from build123d import *

# Parameters (mm, degrees)
EXTRUDE_1_DEPTH     = 10
CUT_EXTRUDE_1_REACH = 177.427
SKETCH_2_R          = 2.15
FILLET_1_R          = 0.6


with BuildPart() as part:
    # 草图1 → 凸台-拉伸1 (new body)
    with BuildSketch(Plane(origin=(0, 0, 0), x_dir=(1, 0, 0), z_dir=(0, 1, 0))):
        with BuildLine():
            Line((-19, 0), (19, 0))
            Line((19, 0), (44.854614973, 30.81233028))
            ThreePointArc((44.854614973, 30.81233028), (46.529317931, 33.929104052), (46.82231051, 37.455159084))
            Line((46.82231051, 37.455159084), (33.389549678, 146.856216784))
            ThreePointArc((33.389549678, 146.856216784), (34.753999407, 148.533855984), (36.376927445, 147.104765038))
            ThreePointArc((36.376927445, 147.104765038), (36.892496808, 144.296291333), (37.320815542, 141.473193853))
            Line((37.320815542, 141.473193853), (37.815132232, 139.258398169))
            ThreePointArc((37.815132232, 139.258398169), (37.817176658, 139.245056143), (37.817405692, 139.231560332))
            Line((37.817405692, 139.231560332), (37.557917484, 134.104765038))
            ThreePointArc((37.557917484, 134.104765038), (40.754926912, 130.959847465), (43.503129215, 134.503681536))
            Line((43.503129215, 134.503681536), (43.077003941, 137.813685213))
            Line((43.077003941, 137.813685213), (42.807637334, 138.925557366))
            ThreePointArc((42.807637334, 138.925557366), (42.806315787, 138.931905108), (42.80540838, 138.938325149))
            Line((42.80540838, 138.938325149), (42.129277547, 145.175318139))
            Line((42.129277547, 145.175318139), (41.965181023, 146.44996701))
            ThreePointArc((41.965181023, 146.44996701), (43.130662006, 148.010841711), (44.727999785, 146.895858405))
            Line((44.727999785, 146.895858405), (66.016482503, 37.376109146))
            ThreePointArc((66.016482503, 37.376109146), (66.063066684, 33.817543133), (64.860464706, 30.468019192))
            Line((64.860464706, 30.468019192), (38.23055697, -15.656334008))
            ThreePointArc((38.23055697, -15.656334008), (35.050772773, -18.836118205), (30.707106781, -20))
            Line((30.707106781, -20), (5.707106781, -20))
            ThreePointArc((5.707106781, -20), (5.515765065, -19.961939766), (5.353553391, -19.853553391))
            Line((5.353553391, -19.853553391), (5, -19.5))
            Line((5, -19.5), (-5, -19.5))
            Line((-5, -19.5), (-5.353553391, -19.853553391))
            ThreePointArc((-5.353553391, -19.853553391), (-5.515765065, -19.961939766), (-5.707106781, -20))
            Line((-5.707106781, -20), (-25.399802658, -20))
            ThreePointArc((-25.399802658, -20), (-30.087775174, -18.833058003), (-33.681629288, -15.604582738))
            Line((-33.681629288, -15.604582738), (-64.860464706, 30.468019192))
            ThreePointArc((-64.860464706, 30.468019192), (-66.063066684, 33.817543133), (-66.016482503, 37.376109146))
            Line((-66.016482503, 37.376109146), (-46.829620455, 141.890886738))
            ThreePointArc((-46.829620455, 141.890886738), (-43.465252598, 152.148967586), (-37.480163066, 161.13372674))
            ThreePointArc((-37.480163066, 161.13372674), (-33.620696298, 161.680216975), (-32.479267504, 157.953116813))
            ThreePointArc((-32.479267504, 157.953116813), (-35.579400499, 146.14570295), (-34.973851142, 133.953116813))
            Line((-34.973851142, 133.953116813), (-47.176674229, 34.569098196))
            ThreePointArc((-47.176674229, 34.569098196), (-47.109221395, 33.75732882), (-46.723670812, 33.03978429))
            Line((-46.723670812, 33.03978429), (-19, 0))
        make_face()
    extrude(amount=EXTRUDE_1_DEPTH)

    # 草图2 → 切除-拉伸1 (cut, up to next)
    with BuildSketch(Plane(origin=(0, 10, 0), x_dir=(1, 0, 0), z_dir=(0, 1, 0)), mode=Mode.PRIVATE) as cut_extrude_1_sk1:
        with Locations(Location((0, -15.5, 0), (0, 0, 270))):
            Circle(SKETCH_2_R)
    cut_extrude_1_tool1 = extrude(cut_extrude_1_sk1.sketch, amount=-CUT_EXTRUDE_1_REACH, mode=Mode.PRIVATE) & part.part
    # 草图2 → 切除-拉伸1 (cut, up to next)
    with BuildSketch(Plane(origin=(0, 10, 0), x_dir=(1, 0, 0), z_dir=(0, 1, 0)), mode=Mode.PRIVATE) as cut_extrude_1_sk2:
        with Locations(Location((0, -7.5, 0), (0, 0, 270))):
            Circle(SKETCH_2_R)
    cut_extrude_1_tool2 = extrude(cut_extrude_1_sk2.sketch, amount=-CUT_EXTRUDE_1_REACH, mode=Mode.PRIVATE) & part.part
    # 草图2 → 切除-拉伸1 (cut, up to next)
    with BuildSketch(Plane(origin=(0, 10, 0), x_dir=(1, 0, 0), z_dir=(0, 1, 0)), mode=Mode.PRIVATE) as cut_extrude_1_sk3:
        with BuildLine():
            Line((-36.549558395, 121.120011078), (-38.607748185, 104.35740041))
            ThreePointArc((-38.607748185, 104.35740041), (-42.47341142, 116.594845153), (-44.332546284, 129.292956179))
            Line((-44.332546284, 129.292956179), (-43.845113062, 129.987442667))
            ThreePointArc((-43.845113062, 129.987442667), (-43.702378092, 130.509625408), (-43.924830211, 131.003146575))
            Line((-43.924830211, 131.003146575), (-44.447419993, 131.543571067))
            ThreePointArc((-44.447419993, 131.543571067), (-44.482588605, 132.737575539), (-44.499925482, 133.931972015))
            ThreePointArc((-44.499925482, 133.931972015), (-41.418283025, 136.952003662), (-38.505677682, 133.768634142))
            ThreePointArc((-38.505677682, 133.768634142), (-38.556072369, 132.542586282), (-38.556286633, 131.315503182))
            Line((-38.556286633, 131.315503182), (-38.546052546, 131.325051295))
            ThreePointArc((-38.546052546, 131.325051295), (-38.780683801, 130.91622187), (-38.744387532, 130.446247504))
            Line((-38.744387532, 130.446247504), (-38.486748585, 129.793872308))
            ThreePointArc((-38.486748585, 129.793872308), (-37.841140795, 125.384806825), (-36.549558395, 121.120011078))
        make_face()
    cut_extrude_1_tool3 = extrude(cut_extrude_1_sk3.sketch, amount=-CUT_EXTRUDE_1_REACH, mode=Mode.PRIVATE) & part.part
    add(cut_extrude_1_tool1.solids().sort_by_distance((0, 10, 15.5))[0], mode=Mode.SUBTRACT)
    add(cut_extrude_1_tool2.solids().sort_by_distance((0, 10, 7.5))[0], mode=Mode.SUBTRACT)
    add(cut_extrude_1_tool3.solids().sort_by_distance((-40.502089, 10, -123.156617))[0], mode=Mode.SUBTRACT)

    # 圆角1
    fillet_1_edges = [part.edges().sort_by_distance(p)[0] for p in [
        (-36.549558395, 5, -121.120011078),
        (-34.973851142, 5, -133.953116813),
    ]]
    fillet(fillet_1_edges, radius=FILLET_1_R)


solid = part.part
The listing builds one solid part. Answer for the finished solid, in the listing's coordinates (mm). A direction names the side the tool comes from. Coordinates: 2 decimals unless noted, no trailing zeros. Write each loop counter-clockwise with the first axis right and the second up, starting at its lowest first coordinate (ties: lowest second). Pieces come first, ordered by that corner, then holes. Notation, with made-up numbers: (43.25, 86.25) - (87.25, 86.25) arc R12 ccw to (87.25, 100.25) - close; hole circle Ø3 at (27.25, -12). An arc over 180 degrees is marked (long way). Return JSON: item names as keys, results as strings.
1. Each of these flat-tipped pins is pushed along its axis until it touches: pin 1 Ø5 at (x, y) = (-0.5, 3.5) entering from -Z; pin 2 Ø6 at (y, z) = (7.5, -115.5) entering from -X; pin 3 Ø3 at (x, y) = (0, 2.5) entering from +Z; pin 4 Ø5.5 at (x, z) = (40.55, -133.95) entering from -Y. Where does it stop, or does it pass through?
Final values:
{"pin 1": "z = 0", "pin 2": "x = -52.23", "pin 3": "z = 19.5", "pin 4": "through"}
2. The part is cut by section B-B on z = -24. Determine the outline of the cut face in (x, y), then the cut area to 3 significant figures.
Final values:
{"outline": "(-60.48, 0) - (-39.14, 0) - (-39.14, 10) - (-60.48, 10) - close; (39.14, 0) - (61.13, 0) - (61.13, 10) - (39.14, 10) - close", "area": "433 mm^2"}
3. The part is cut by section A-A on x = 0. Determine the outline of the cut face in (y, z).
Final values:
{"outline": "(0, 0) - (10, 0) - (10, 5.35) - (0, 5.35) - close; (0, 9.65) - (10, 9.65) - (10, 13.35) - (0, 13.35) - close; (0, 17.65) - (10, 17.65) - (10, 19.5) - (0, 19.5) - close"}
4. Consider line 1 along X through (y, z) = (9, -143.5); line 2 along X through (y, z) = (8.75, -126); line 3 along Z through (x, y) = (-13.5, 3.5). Determine where each line is inside the solid, lowest interval first.
Final values:
{"line 1": "-46.5 to -35.77, 33.8 to 37.02, 42.31 to 45.39", "line 2": "-49.75 to -44.05, -37.97 to -35.95, 35.95 to 48.79", "line 3": "0 to 20"}
5. The part is cut by section C-C on y = 1.75. Count the separate pieces of the cut face and the enclosed holes in it, then the cut area to 3 significant figures.
Final values:
{"separate pieces": "1", "enclosed holes": "2", "area": "6,520 mm^2"}
6. For a pull along Z with two mould halves and no side action, classify faces 4 (the face through (-41.486, 5.07, -136.953)), 5 (the face through (-15, 5, 20)), 6 (the face through (0, 5, 0)) as +Z half, -Z half, draft (parallel to the pull), parting line (faces both ways), or undercut.
Final values:
{"face 4": "undercut", "face 5": "+Z half", "face 6": "-Z half"}
7. The part is cut by section D-D on z = -51. Determine the outline of the cut face in (x, y), then the cut area to 3 significant figures.
Final values:
{"outline": "(-63.52, 0) - (-45.16, 0) - (-45.16, 10) - (-63.52, 10) - close; (45.16, 0) - (63.37, 0) - (63.37, 10) - (45.16, 10) - close", "area": "366 mm^2"}
8. Which of the six approach directions +Z, -Z, +X, -X, +Y, -Y give full straight-line access (tool end or side, diameter ignored) to faces 1 (the face through (0, 5, 19.5)), 2 (the face through (37.69, 4.93, -136.7)), 3 (the face through (35.11, 4.93, 18.8))?
Final values:
{"face 1": "+Z, +Y, -Y", "face 2": "+Y, -Y", "face 3": "+Z, +X, +Y, -Y"}
